The drawing under review shows one solid part. Ordinate dimensions are in mm from its lowest x, y, z. A direction names the side the tool comes from. Round coordinates to 2 decimals unless told otherwise and drop trailing zeros. Order: outer loops, then holes, each group sorted by start corner. A loop starts at its lowest first (then second) coordinate and runs counter-clockwise, first axis right, second up. Notation, with made-up numbers: (79, 39) -> (131, 39) arc R7 ccw to (131, 52) -> close; hole circle Ø8 at (-13.5, 32.25). An arc over 180 degrees is marked (long way). Return JSON: item names as keys, results as strings. Group by question number.
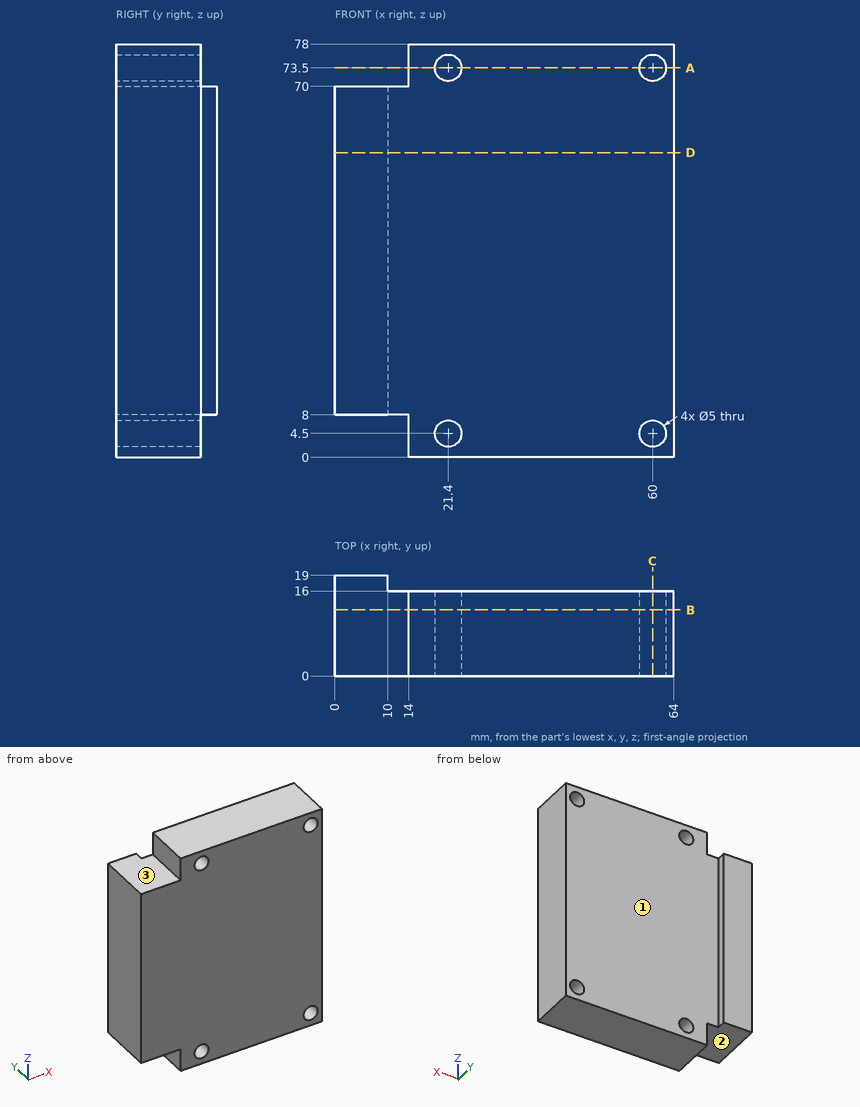
Item 1: Consider section B-B on y = 12.5. State the section outline as (x, z) points, plus the area to 3 significant figures.
Item 2: Consider section D-D on z = 57.5. State the section outline as (x, y) points.
Item 3: For the marked faces 1, 2 and 3, list the 3-axis set-ups (+Z, -Z, +X, -X, +Y, -Y) from which the entire face can be reached by the end or side of a thin tool; tool diameter is ignored.
Item 4: Consider section C-C on x = 60. State the section outline as (y, z) points.
Item 5: Insertion check: pin 1 Ø1.5 at (y, z) = (17, 45) entering from +X; pin 2 Ø4 at (x, y) = (7.5, 14) entering from -Z; pin 3 Ø3 at (x, z) = (21.4, 4.5) entering from -Y; pin 4 Ø4 at (x, y) = (8.5, 6.5) entering from +Z. Each pin has a flat end and moves straight along its axis. Give the tip position at first contact, or say it passes through.
Item 6: Wall thickness on line 1 along X through (y, z) = (6.75, 4.5); line 2 along X through (y, z) = (7.75, 75.5); line 3 along Z through (x, y) = (22, 1): over which ranges is each line inside the solid? List them lowest first.
Item 7: Consider section A-A on z = 73.5. State the section outline as (x, y) points.
Values:
{
 "1": {"outline": "(0, 8) -> (14, 8) -> (14, 0) -> (64, 0) -> (64, 78) -> (14, 78) -> (14, 70) -> (0, 70) -> close; hole circle Ø5 at (21.4, 4.5); hole circle Ø5 at (21.4, 73.5); hole circle Ø5 at (60, 4.5); hole circle Ø5 at (60, 73.5)", "area": "4,690 mm^2"},
 "2": {"outline": "(0, 0) -> (64, 0) -> (64, 16) -> (10, 16) -> (10, 19) -> (0, 19) -> close"},
 "3": {"face 1": "+Z, -Z, +X, +Y", "face 2": "-Z, -X, +Y, -Y", "face 3": "+Z, -X, +Y, -Y"},
 "4": {"outline": "(0, 0) -> (16, 0) -> (16, 2) -> (0, 2) -> close; (0, 7) -> (16, 7) -> (16, 71) -> (0, 71) -> close; (0, 76) -> (16, 76) -> (16, 78) -> (0, 78) -> close"},
 "5": {"pin 1": "x = 10", "pin 2": "z = 8", "pin 3": "through", "pin 4": "z = 70"},
 "6": {"line 1": "14 to 18.9, 23.9 to 57.5, 62.5 to 64", "line 2": "14 to 19.9, 22.9 to 58.5, 61.5 to 64", "line 3": "0 to 2.07, 6.93 to 71.07, 75.93 to 78"},
 "7": {"outline": "(14, 0) -> (18.9, 0) -> (18.9, 16) -> (14, 16) -> close; (23.9, 0) -> (57.5, 0) -> (57.5, 16) -> (23.9, 16) -> close; (62.5, 0) -> (64, 0) -> (64, 16) -> (62.5, 16) -> close"}
}
